```python
from build123d import *

# Parameters (mm, degrees)
CYLINDER002_R     = 28.3
CYLINDER002_DEPTH = 42
BOX004_W          = 42
BOX004_H          = 56.6
BOX004_DEPTH      = 52


with BuildPart() as top_cylinder001:
    # Cylinder002 → Cylinder002 (new body)
    with BuildSketch(Plane(origin=(-2, -6.5, 0), x_dir=(0, 0, -1), z_dir=(1, 0, 0))):
        Circle(CYLINDER002_R)
    extrude(amount=CYLINDER002_DEPTH)


with BuildPart() as bisect_intersect:
    # Box004 → Box004 (new body)
    with BuildSketch(Plane(origin=(-2, 21.8, 0), x_dir=(1, 0, 0), z_dir=(0, 0, -1))):
        with Locations((21, 28.3)):
            Rectangle(BOX004_W, BOX004_H)
    extrude(amount=BOX004_DEPTH)

    # Fusion002: union top cylinder001
    add(top_cylinder001.part)


solid = bisect_intersect.part
```
Input: part model. Units: mm. Frame: model coordinates. Coordinates: 2 decimals unless noted, no trailing zeros. Write each loop counter-clockwise with the first axis right and the second up, starting at its lowest first coordinate (ties: lowest second). Pieces come first, ordered by that corner, then holes. Notation, with made-up numbers: (-6, 87) -> (19, 87) arc R12 ccw to (19, 100) -> close; hole circle Ø11 at (20, 30). An arc over 180 degrees is marked (long way). Answer as a JSON object with one key per item and string values.
1. First-contact query: P1, Ø5, axis at x = 19, y = 11.5, coming from the +Z side; P2, Ø2, axis at x = 21.5, y = -22, coming from the +Z side; P3, Ø2, axis at x = 22.5, z = 8.5, coming from the -Y side. Flat tips, straight axial feed; report the tip coordinate or a pass-through.
Result set:
{"P1": "stops at z = 23.68", "P2": "stops at z = 24.3", "P3": "stops at y = -33.79"}
2. Section A-A on z = 20.5. Return the cut outline in (x, y).
Result set:
{"outline": "(-2, -26.01) -> (40, -26.01) -> (40, 13.01) -> (-2, 13.01) -> close"}
3. Material intervals for line 1 (Z direction, x = 18, y = -7); line 2 (Z direction, x = 27, y = 12.5); line 3 (Y direction, x = 15.5, z = 21.5), sorted ascending. Write a range as from..to.
Result set:
{"line 1": "z = -52..28.3", "line 2": "z = -52..20.97", "line 3": "y = -24.9..11.9"}
4. Section B-B on x = 25.5. Return the cut outline in (y, z), then the cut area to 3 significant figures.
Result set:
{"outline": "(-34.8, -52) -> (21.8, -52) -> (21.8, 0) arc R28.3 ccw to (-34.8, 0) -> close", "area": "4,200 mm2"}
